from build123d import *

# Parameters (mm, degrees)
BOSS_EXTRUDE5_DEPTH = 150
SKETCH6_W           = 101.090693468
SKETCH6_H           = 50
SKETCH6_H_2         = 500
CUT_EXTRUDE1_DEPTH  = 654.146231712
CUT_EXTRUDE2_REACH  = 655.146
SKETCH7_W           = 160
SKETCH7_H           = 150
SKETCH8_W           = 48.75
SKETCH8_H           = 19
BOSS_EXTRUDE6_DEPTH = 19
BOSS_EXTRUDE8_DEPTH = 19


with BuildPart() as part:
    # Sketch5 → Boss-Extrude5 (new body)
    with BuildSketch(Plane.XY):
        Polygon((0, 600), (0, 0), (25, 0), (25, 575), (185, 575), (185, 0), (210, 0), (210, 600), align=None)
    extrude(amount=BOSS_EXTRUDE5_DEPTH)

    # Sketch6 → Cut-Extrude1 (cut, through all)
    with BuildSketch(Plane.ZY):
        with Locations((75, 25)):
            Rectangle(SKETCH6_W, SKETCH6_H)
        with Locations((75, 325)):
            Rectangle(SKETCH6_W, SKETCH6_H_2)
    extrude(amount=-CUT_EXTRUDE1_DEPTH, mode=Mode.SUBTRACT)

    # Sketch7 → Cut-Extrude2 (cut, up to next)
    with BuildSketch(Plane(origin=(0, 600, 0), x_dir=(1, 0, 0), z_dir=(0, 1, 0)), mode=Mode.PRIVATE) as cut_extrude2_sk1:
        with Locations((105, -75)):
            Rectangle(SKETCH7_W, SKETCH7_H)
    cut_extrude2_tool1 = extrude(cut_extrude2_sk1.sketch, amount=-CUT_EXTRUDE2_REACH, mode=Mode.PRIVATE) & part.part
    add(cut_extrude2_tool1.solids().sort_by_distance((105, 600, 75))[0], mode=Mode.SUBTRACT)


with BuildPart() as cut_extrude2_piece_1:
    # of the separate pieces the step leaves, piece 1, a body of its own (cut_extrude2_pieces)
    add(part.part.solids().sort_by_distance((0, 600, 0))[0])

    # Sketch8 → Boss-Extrude6 (add)
    with BuildSketch(Plane(origin=(0, 0, 0), x_dir=(-1, 0, 0), z_dir=(0, 0, -1))):
        with Locations((-160.625, 520.5)):
            Rectangle(SKETCH8_W, SKETCH8_H)
        with Locations((-49.375, 520.5)):
            Rectangle(SKETCH8_W, SKETCH8_H)
    extrude(amount=-BOSS_EXTRUDE6_DEPTH)


with BuildPart() as cut_extrude2_piece_2:
    # of the separate pieces the step leaves, piece 2, a body of its own (cut_extrude2_pieces)
    add(part.part.solids().sort_by_distance((210, 600, 0))[0])



with BuildPart() as boss_extrude6_piece_1:
    # of the separate pieces the step leaves, piece 1, a body of its own (boss_extrude6_pieces)
    add(cut_extrude2_piece_1.part.solids().sort_by_distance((0, 600, 0))[0])


with BuildPart() as boss_extrude6_piece_2:
    # of the separate pieces the step leaves, piece 2, a body of its own (boss_extrude6_pieces)
    add(cut_extrude2_piece_1.part.solids().sort_by_distance((136.25, 530, 0))[0])


with BuildPart() as cut_extrude2_piece_2_1:
    add(cut_extrude2_piece_2.part)

    add(boss_extrude6_piece_1.part)  # Boss-Extrude8 merges Boss-Extrude6 piece 1

    add(boss_extrude6_piece_2.part)  # Boss-Extrude8 merges Boss-Extrude6 piece 2
    # Sketch10 → Boss-Extrude8 (add)
    with BuildSketch(Plane(origin=(0, 530, 0), x_dir=(1, 0, 0), z_dir=(0, 1, 0))):
        Polygon((185, -150), (25, -150), (25, -131), (54.75, -131), (54.75, -19), (73.75, -19), (73.75, -131), (136.25, -131), (136.25, -19), (155.25, -19), (155.25, -131), (185, -131), align=None)
    extrude(amount=-BOSS_EXTRUDE8_DEPTH)


solid = cut_extrude2_piece_2_1.part
Geometry check sheet. Reference: the model listing, model coordinates, mm. A direction names the side the tool comes from. Round coordinates to 2 decimals unless told otherwise and drop trailing zeros. Write each loop counter-clockwise with the first axis right and the second up, starting at its lowest first coordinate (ties: lowest second). Pieces come first, ordered by that corner, then holes. Notation, with made-up numbers: (-37.5, 14) - (6.5, 14) arc R25 ccw to (6.5, 45) - close; hole circle Ø10 at (89, 57). An arc over 180 degrees is marked (long way). One line per item, written item: value.
1. Scan lines: L1, parallel to Y at x = 196, z = 60; L2, parallel to X at y = 529, z = 102; L3, parallel to X at y = 551, z = 138. Record each from-to range of solid material in increasing order.
The answers:
L1: y = 50 to 75, 575 to 600
L2: x = 54.75 to 73.75, 136.25 to 155.25
L3: x = 0 to 25, 185 to 210
2. Cross-section at D-D on x = 101. Record the boundary of the cut face in (y, z), and give its area (3 significant figures).
The answers:
outline: (511, 131) - (530, 131) - (530, 150) - (511, 150) - close
area: 361 mm^2
3. Mould release check, pull along Z, two halves, no side actions. Record for faces 6 (the face through (105, 521, 131)), 7 (the face through (155.25, 521, 74)), 8 (the face through (12, 0, 138)): released by +Z, released by -Z, zero draft, split by the parting line, or undercut.
The answers:
face 6: released by -Z
face 7: undercut
face 8: zero draft
4. Cross-section at C-C on z = 33.5. Record the boundary of the cut face in (x, y).
The answers:
outline: (0, 50) - (25, 50) - (25, 75) - (0, 75) - close; (0, 575) - (25, 575) - (25, 600) - (0, 600) - close; (54.75, 511) - (73.75, 511) - (73.75, 530) - (54.75, 530) - close; (136.25, 511) - (155.25, 511) - (155.25, 530) - (136.25, 530) - close; (185, 50) - (210, 50) - (210, 75) - (185, 75) - close; (185, 575) - (210, 575) - (210, 600) - (185, 600) - close
5. Set-up check for faces 1 (the face through (141, 511, 91)), 2 (the face through (197, 75, 74)), 3 (the face through (170, 521, 131)), 4 (the face through (197, 25, 24.455)), 5 (the face through (136.25, 521, 66)): record each of +Z, -Z, +X, -X, +Y, -Y from which the full face is reachable in a straight line by a thin tool's end or side.
The answers:
face 1: +Z, -Z, -Y
face 2: +X, -X
face 3: +Y, -Y
face 4: +X, -X, -Y
face 5: -Z, +Y, -Y
6. Depth check by flat-ended pin: pin 1 Ø15 at (y, z) = (521.5, 73) entering from -X; pin 2 Ø7.5 at (x, z) = (201, 83.5) entering from -Y; pin 3 Ø8 at (x, z) = (77.5, 133) entering from -Y. Enter the tip coordinate at first touch or a pass-through.
The answers:
pin 1: stops at x = 54.75
pin 2: stops at y = 50
pin 3: stops at y = 511
7. Cross-section at B-B on x = 196. Record the boundary of the cut face in (y, z).
The answers:
outline: (0, 0) - (600, 0) - (600, 150) - (0, 150) - (0, 125.55) - (50, 125.55) - (50, 24.45) - (0, 24.45) - close; hole (75, 24.45) - (575, 24.45) - (575, 125.55) - (75, 125.55) - close
8. Cross-section at A-A on y = 40.5. Record the boundary of the cut face in (x, z), and give its area (3 significant figures).
The answers:
outline: (0, 0) - (25, 0) - (25, 24.45) - (0, 24.45) - close; (0, 125.55) - (25, 125.55) - (25, 150) - (0, 150) - close; (185, 0) - (210, 0) - (210, 24.45) - (185, 24.45) - close; (185, 125.55) - (210, 125.55) - (210, 150) - (185, 150) - close
area: 2,450 mm^2
